```python
from build123d import *

# Parameters (mm, degrees)
SKETCH_1_R          = 1
EXTRUDE_1_DEPTH     = 3
SKETCH_4_R          = 0.8
SKETCH_4_R_2        = 1.65
CUT_EXTRUDE_2_DEPTH = 18
SKETCH_6_W          = 178.5
SKETCH_6_H          = 1
EXTRUDE_2_DEPTH     = 3


with BuildPart() as part:
    # 草图1 → 凸台-拉伸1 (new body)
    with BuildSketch(Plane(origin=(0, 0, 0), x_dir=(1, 0, 0), z_dir=(0, 1, 0))):
        with BuildLine():
            Line((-150, 40), (71, 40))
            ThreePointArc((71, 40), (126.861435714, 16.861435714), (150, -39))
            Line((150, -39), (150, -40))
            Line((150, -40), (-150, -40))
            Line((-150, -40), (-150, 40))
        make_face()
        with Locations(Location((-117.057778193, 37, 0), (0, 0, 270))):
            Circle(SKETCH_1_R, mode=Mode.SUBTRACT)
        with Locations(Location((-147.557778193, 37, 0), (0, 0, 270))):
            Circle(SKETCH_1_R, mode=Mode.SUBTRACT)
        with Locations(Location((-147.557778193, -3, 0), (0, 0, 270))):
            Circle(SKETCH_1_R, mode=Mode.SUBTRACT)
    extrude(amount=EXTRUDE_1_DEPTH)

    # 草图4 → 切除-拉伸2 (cut)
    with BuildSketch(Plane(origin=(0, 0, 0), x_dir=(1, 0, 0), z_dir=(0, 1, 0))):
        Polygon((-34, 2.44312071), (62.924700675, 34), (-34, 34), align=None)
        Polygon((68.5, -27.5), (68.5, 30.55687929), (-28.424700675, -1), (54.5, -27.998739755), (54.5, -27.5), align=None)
        Polygon((-39, 2.44312071), (-39, 34), (-135.924700675, 34), align=None)
        with Locations(Location((68, -34.5, 0), (0, 0, 270))):
            Circle(SKETCH_4_R)
        Polygon((54.5, -36), (54.5, -33.257074199), (-34, -4.44312071), (-34, -36), align=None)
        Polygon((-125.968156468, -27.5), (-44.575299325, -1), (-144, 31.370832778), (-144, -27.5), align=None)
        Polygon((-39, -36), (-39, -4.44312071), (-124, -32.117539315), (-124, -36), align=None)
        with BuildLine():
            Line((73.5, 28.585131501), (73.5, -36))
            Line((73.5, -36), (138.527772065, -36))
            ThreePointArc((138.527772065, -36), (142.265497073, -34.321055821), (143.493049422, -30.411764706))
            ThreePointArc((143.493049422, -30.411764706), (122.427421924, 12.809461243), (79.051470588, 33.554626464))
            ThreePointArc((79.051470588, 33.554626464), (75.165135156, 32.310541072), (73.5, 28.585131501))
        make_face()
        with Locations(Location((-129.5, -34.5, 0), (0, 0, 270))):
            Circle(SKETCH_4_R)
        with Locations(Location((-135.5, -34.5, 0), (0, 0, 270))):
            Circle(SKETCH_4_R)
        with Locations(Location((62, -34.5, 0), (0, 0, 270))):
            Circle(SKETCH_4_R)
        with Locations((-144, 40)):
            Circle(SKETCH_4_R_2)
    extrude(amount=CUT_EXTRUDE_2_DEPTH, mode=Mode.SUBTRACT)

    # 草图6 → 凸台-拉伸2 (add, through all)
    with BuildSketch(Plane(origin=(0, 3, 0), x_dir=(1, 0, 0), z_dir=(0, 1, 0))):
        with Locations((-34.75, -35.5)):
            Rectangle(SKETCH_6_W, SKETCH_6_H)
    extrude(amount=-EXTRUDE_2_DEPTH)


solid = part.part
```
Input: part model. Units: mm. Frame: model coordinates. A direction names the side the tool comes from. Give positions to 0.01 mm unless a question says otherwise; leave off trailing zeros. Loops run counter-clockwise (first coordinate to the right, second up) from the corner with the lowest first, then second, coordinate; pieces in that order, holes last.
1) Section query C-C on x = 15. Return the cut outline in (y, z).
A:
outline: (0, -40) - (3, -40) - (3, -34) - (0, -34) - close; (0, -18.4) - (3, -18.4) - (3, -13.14) - (0, -13.14) - close; (0, 15.14) - (3, 15.14) - (3, 20.4) - (0, 20.4) - close; (0, 35) - (3, 35) - (3, 40) - (0, 40) - close
2) Section query D-D on y = 1.95. Count the separate pieces of the cut face and the enclosed holes in it, and give its area (3 significant figures).
A:
separate pieces: 1
enclosed holes: 14
area: 6,770 mm2
3) Mould query, pull axis Z, two halves, no side actions, for faces 3 (the flat face through (13.78, 1.48, -18)), 4 (the cylindrical face through (126.244, 1.479, -17.472)), 5 (the flat face through (-23, 0, 6)). Classes: released by +Z, released by -Z, zero draft, split by the parting line, or undercut.
A:
face 3: undercut
face 4: released by -Z
face 5: zero draft
4) Line query: L1, parallel to Z at x = 2.5, y = 0.9; L2, parallel to Z at x = 48, y = 2.7; L3, parallel to Z at x = -30, y = 2.2. Output: solid intervals per line, ascending.
A:
L1: z = -40 to -34, -14.33 to -9.07, 11.07 to 16.33, 35 to 40
L2: z = -40 to -34, -29.14 to -23.88, 25.88 to 31.14, 35 to 40
L3: z = -40 to -34, -3.75 to 5.75, 35 to 40
5) Section query B-B on z = 21. Return the cut outline in (x, y), and give its area (3 significant figures).
A:
outline: (-150, 0) - (-144, 0) - (-144, 3) - (-150, 3) - close; (-106, 0) - (-89.85, 0) - (-89.85, 3) - (-106, 3) - close; (-39, 0) - (-34, 0) - (-34, 3) - (-39, 3) - close; (16.85, 0) - (33, 0) - (33, 3) - (16.85, 3) - close; (68.5, 0) - (73.5, 0) - (73.5, 3) - (68.5, 3) - close; (141.75, 0) - (147.92, 0) - (147.92, 3) - (141.75, 3) - close
area: 163 mm2
6) Reachability of faces 1 (the flat face through (12.46, 1.48, 14.31)), 2 (the flat face through (-23, 3, 6)) from +Z, -Z, +X, -X, +Y, -Y: full face, straight path, thin tool, end or side. Return the list, or none.
A:
face 1: +Y, -Y
face 2: +Z, -Z, +X, -X, +Y
7) Section query A-A on x = 99.5. Return the cut outline in (y, z), and give its area (3 significant figures).
A:
outline: (0, -34.68) - (3, -34.68) - (3, -28.21) - (0, -28.21) - close; (0, 36) - (3, 36) - (3, 40) - (0, 40) - close
area: 31.4 mm2
8) Contact query for flat-ended pins moving along their axis: pin 1 (1 mm diameter, centred on y = 2, z = -21, fed in from +X); pin 2 (0.9 mm diameter, centred on y = 2, z = 9, fed in from +X). Output: stop coordinate, or through.
A:
pin 1: stops at x = 122.97
pin 2: stops at x = 144.27
